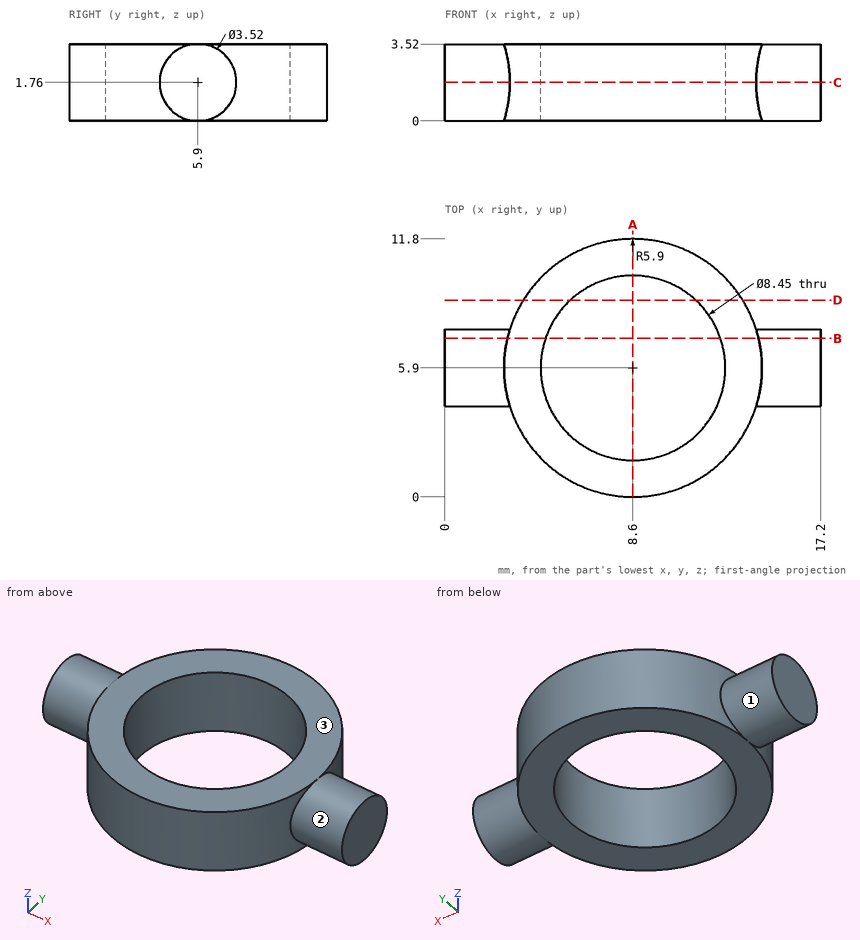
Here's the drawing with two shaded views (mm, measured from the low corner). I have some questions. A direction names the side the tool comes from. Coordinates: 2 decimals unless noted, no trailing zeros. Write each loop counter-clockwise with the first axis right and the second up, starting at its lowest first coordinate (ties: lowest second). Pieces come first, ordered by that corner, then holes. Notation, with made-up numbers: M -15.5,75.5 L 34.5,75.5 A13 cw 34.5,91.5 Z; hole C -24.5,-12.5 d8. An arc over 180 degrees is marked long. Answer as CSV lines item,"result". Start each with the question number.
1) Please list where these lines run through material, in increasing order: line 1 (X direction, y = 8.5, z = 1.5); line 2 (X direction, y = 6.25, z = 1.4); line 3 (Y direction, x = 6.75, z = 1.6). Write a range as from..to.
2) For P1, Ø1, axis at y = 10.5, z = 2, coming from the -X side; P2, Ø2, axis at x = 5, z = 2.5, coming from the -Y side, each with a flat end and sliding along its axis, tell me the tip position at first contact or that it passes through.
3) I want a section at C-C, the plane z = 1.76. Please give me the cut outline in (x, y) (3 decimals), and give its area (3 significant figures).
4) I want a section at D-D, the plane y = 9. Please give me the cut outline in (x, z).
5) I want a section at B-B, the plane y = 7.25. Please give me the cut outline in (x, z).
6) For the marked faces 1, 2 and 3, which set-ups out of +Z, -Z, +X, -X, +Y, -Y let a thin tool reach every point of the face, with its end or its side?
7) I want a section at A-A, the plane x = 8.6. Please give me the cut outline in (y, z) (3 decimals).
Data:
1,line 1,"x = 3.3..5.27, 11.93..13.9"
1,line 2,"x = 0..4.39, 12.81..17.2"
1,line 3,"y = 0.3..2.1, 9.7..11.5"
2,P1,"stops at x = 4.36"
2,P2,"stops at y = 0.6"
3,outline,"M 0,4.14 L 2.969,4.14 A5.9 ccw 14.231,4.14 L 17.2,4.14 L 17.2,7.66 L 14.231,7.66 A5.9 ccw 2.969,7.66 L 0,7.66 Z; hole C 8.6,5.9 d8.45"
3,area,"72.9 mm^2"
4,outline,"M 3.58,0 L 5.73,0 L 5.73,3.52 L 3.58,3.52 Z; M 11.47,0 L 13.62,0 L 13.62,3.52 L 11.47,3.52 Z"
5,outline,"M 0,0.63 L 2.86,0.63 L 2.86,0 L 4.6,0 L 4.6,3.52 L 2.86,3.52 L 2.86,2.89 L 0,2.89 Z; M 12.6,0 L 14.34,0 L 14.34,0.63 L 17.2,0.63 L 17.2,2.89 L 14.34,2.89 L 14.34,3.52 L 12.6,3.52 Z"
6,face 1,"-X"
6,face 2,"+X"
6,face 3,"+Z, +X, -X, +Y, -Y"
7,outline,"M 0,0 L 1.675,0 L 1.675,3.52 L 0,3.52 Z; M 10.125,0 L 11.8,0 L 11.8,3.52 L 10.125,3.52 Z"
